Geometry: final body of the model. Coordinates: model frame, mm. Give positions to 0.01 mm unless a question says otherwise; leave off trailing zeros. Write each loop counter-clockwise with the first axis right and the second up, starting at its lowest first coordinate (ties: lowest second). Pieces come first, ordered by that corner, then holes. Notation, with made-up numbers: M 15.5,-1 L 19.5,-1 A14 cw 19.5,12 Z; hole C -16.75,65 d7. An arc over 180 degrees is marked long. Use one line per item in the form item = value. Start each with the question number.
Item 1: Contact query for flat-ended pins moving along their axis: P1, Ø10, axis at x = 62.5, y = 39, coming from the +Z side; P2, Ø1, axis at x = 47, z = 1, coming from the +Y side; P3, Ø0.6, axis at y = 91, z = 1.5, coming from the -X side. Output: stop coordinate, or through.
Item 2: Material intervals for line 1 along X through (y, z) = (86.5, 2.2); line 2 along Z through (x, y) = (38.5, 17.5), sorted ascending. Write a range as from..to.
Item 3: Section query B-B on x = 39. Return loops of the section in (y, z), then the cut area to 3 significant figures.
Item 4: Section query A-A on y = 56. Return loops of the section in (x, z).
Item 5: Pull-direction query (X, two-part tool) for faces 1 (the flat face through (37, 68, 0)), 2 (the flat face through (37, 69, 1)); classes: released by +X, released by -X, zero draft, split by the parting line, or undercut.
from build123d import *

# Parameters (mm, degrees)
F1_DEPTH     = 3
F0_W         = 73
F0_H         = 134
F2_DEPTH     = 1
F3_T1_DEPTH  = 145
F3_T3_DEPTH  = 85
F4_T1_DEPTH  = 6
F4_S5_W      = 2
F4_S5_H      = 2
F4_T6_DEPTH  = 2
F4_S11_W     = 2
F4_S11_H     = 2
F4_T12_DEPTH = 2


# Not quite as in the source:
# - a fillet or chamfer that OpenCascade refuses, or shapes differently, is made with other operations: its cross-section is extruded or revolved along the edge and cut away or added


with BuildPart() as f1:
    # F0 (on Top) → F1 (new body)
    with BuildSketch(Plane.XY):
        Polygon((0, 135), (0, 0), (75, 0), (75, 135), (74, 135), (74, 1), (1, 1), (1, 135), align=None)
    extrude(amount=F1_DEPTH)

    # F0 (on Top) → F2 (join)
    with BuildSketch(Plane.XY):
        with Locations((37.5, 68)):
            Rectangle(F0_W, F0_H)
    extrude(amount=F2_DEPTH)

    # F3: fillet of radius 2 on 4 edges, made by hand

    # F3_s2 → F3_t1 (cut)
    with BuildSketch(Plane.XZ.offset(-140)):
        with BuildLine():
            ThreePointArc((0, 2), (0.5857864376, 0.5857864376), (2, 0))
            Line((2, 0), (0, 0))
            Line((0, 0), (0, 2))
        make_face()
        with BuildLine():
            ThreePointArc((75, 2), (74.4142135624, 0.5857864376), (73, 0))
            Line((73, 0), (75, 0))
            Line((75, 0), (75, 2))
        make_face()
    extrude(amount=F3_T1_DEPTH, mode=Mode.SUBTRACT)

    # F3_s4 → F3_t3 (cut)
    with BuildSketch(Plane.YZ.offset(-5)):
        with BuildLine():
            ThreePointArc((2, 0), (0.5857864376, 0.5857864376), (0, 2))
            Line((0, 2), (0, 0))
            Line((0, 0), (2, 0))
        make_face()
        with BuildLine():
            ThreePointArc((133, 0), (134.4142135624, 0.5857864376), (135, 2))
            Line((135, 2), (135, 0))
            Line((135, 0), (133, 0))
        make_face()
    extrude(amount=F3_T3_DEPTH, mode=Mode.SUBTRACT)

    # F4: fillet of radius 2 on 2 edges, made by hand

    # F4_s2 → F4_t1 (cut)
    with BuildSketch(Plane.XY.offset(2)):
        with BuildLine():
            ThreePointArc((73, 0), (74.4142135624, 0.5857864376), (75, 2))
            Line((75, 2), (75, 0))
            Line((75, 0), (73, 0))
        make_face()
        with BuildLine():
            ThreePointArc((0, 2), (0.5857864376, 0.5857864376), (2, 0))
            Line((2, 0), (0, 0))
            Line((0, 0), (0, 2))
        make_face()
    extrude(amount=F4_T1_DEPTH, mode=Mode.SUBTRACT)


with BuildPart() as f4_tool4:
    # F4_s5 → F4_t6 (new body)
    with BuildSketch(Plane.YZ.offset(2)):
        with Locations((1, 1)):
            Rectangle(F4_S5_W, F4_S5_H)
    extrude(amount=-F4_T6_DEPTH)

    # F4_s7 → F4_t8 (revolve, cut)
    with BuildSketch(Plane(origin=(2, 2, 2), x_dir=(0, 0.7071067812, 0.7071067812), z_dir=(0, -0.7071067812, 0.7071067812))):
        with BuildLine():
            ThreePointArc((0, -2), (2, 0), (0, 2))
            Line((0, 2), (0, -2))
        make_face()
    revolve(axis=Axis((2, 2, 2), (-1, 0, 0)), mode=Mode.SUBTRACT)


with BuildPart() as f1_1:
    add(f1.part)

    # F4_t3: cut F4_tool4
    add(f4_tool4.part, mode=Mode.SUBTRACT)


with BuildPart() as f4_tool10:
    # F4_s11 → F4_t12 (new body)
    with BuildSketch(Plane.XZ.offset(-2)):
        with Locations((74, 1)):
            Rectangle(F4_S11_W, F4_S11_H)
    extrude(amount=F4_T12_DEPTH)

    # F4_s13 → F4_t14 (revolve, cut)
    with BuildSketch(Plane(origin=(73, 2, 2), x_dir=(-0.7071067812, 0, 0.7071067812), z_dir=(0.7071067812, 0, 0.7071067812))):
        with BuildLine():
            ThreePointArc((0, -2), (2, 0), (0, 2))
            Line((0, 2), (0, -2))
        make_face()
    revolve(axis=Axis((73, 2, 2), (0, -1, 0)), mode=Mode.SUBTRACT)


with BuildPart() as f1_2:
    add(f1_1.part)

    # F4_t9: cut F4_tool10
    add(f4_tool10.part, mode=Mode.SUBTRACT)


solid = f1_2.part
Answer sheet:
q1.P1 = 1
q1.P2 = 134.73
q1.P3 = 0.01
q2.line_1 = 0..1, 74..75
q2.line_2 = 0..1
q3.outline = M 0,2 A2 ccw 2,0 L 133,0 A2 ccw 134.73,1 L 1,1 L 1,3 L 0,3 Z
q3.area = 135 mm2
q4.outline = M 0,2 A2 ccw 2,0 L 73,0 A2 ccw 75,2 L 75,3 L 74,3 L 74,1 L 1,1 L 1,3 L 0,3 Z
q5.face_1 = zero draft
q5.face_2 = undercut
